The model under review builds one solid part; all positions refer to its coordinate system, in mm. Face numbers are marked on the shaded views. Round coordinates to 2 decimals unless told otherwise and drop trailing zeros. Write each loop counter-clockwise with the first axis right and the second up, starting at its lowest first coordinate (ties: lowest second). Pieces come first, ordered by that corner, then holes.
Item 1: Add section B-B (y = 2.4). Give the boundary of the cut face in (x, z), plus the area to 3 significant figures.
Item 2: Draft analysis for pull direction Z (two halves, no side actions). For the marked faces 1 and 2, state which applies: +Z half, -Z half, draft (parallel to the pull), parting line (faces both ways), or undercut.
Item 3: Clearance check with flat-ended pins moving along their axes: pin 1 Ø2 at (x, z) = (-5.5, -6.5) entering from -Y (3 decimals); pin 2 Ø2 at (x, z) = (-5.5, -8.5) entering from -Y; pin 3 Ø5 at (x, z) = (-12.82, 7.55) entering from +Y; pin 4 Ø1.5 at (x, y) = (4.5, 2.5) entering from -Z. State where each tip first meets the part, or that it passes through.
Item 4: To check wall thickness, follow L1, parallel to X at y = 0.75, z = 0; L2, parallel to Z at x = 0, y = 1.95; L3, parallel to Z at x = 1, y = 2.15. State the ranges of each line that lie inside material, in increasing order.
Item 5: Add section A-A (z = 0). Give the boundary of the cut face in (x, y), plus the area to 3 significant figures.
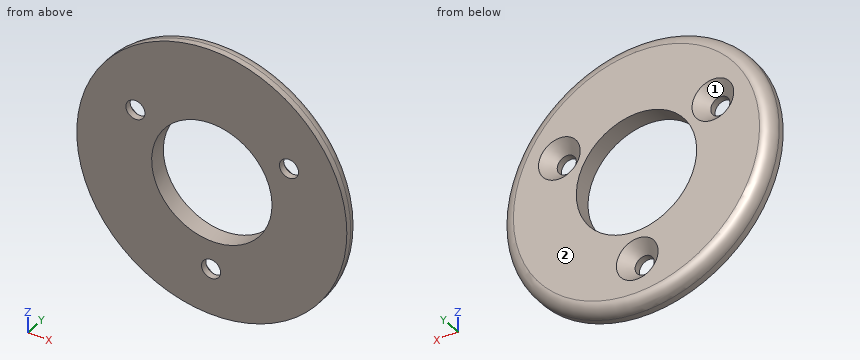
Autodesk Fusion 360 part; units mm, degrees
sketch "Sketch1" plane through (0, 0, 0) normal (0, 1, 0) x (1, 0, 0)
  circle A0 centre (0, 0) radius 22.661
extrude "Extrude1" add sketch "Sketch1" along normal blind 3
hole "Hole1" at (0, 3, 0) direction (0, -1, 0) diameter 20.2 depth 3 tip angle 180
hole "Hole2" at (-0.1263, 3, -14.8781) direction (0, -1, 0) diameter 3.2 depth 30 tip angle 180 countersink diameter 7 countersink angle 90
sketch "Sketch2" plane through (0, 0, 0) normal (0, 1, 0) x (1, 0, 0)
  circle A0 centre (0, 0) radius 15
  dimension "d9" = 30
pattern_circular "C-Pattern1" count 3 over 360 about axis through (0, 0, 0) along (0, 1, 0) of "Hole2"
fillet "Fillet1" radius 2 1 edges at (-21.1274, 3, 8.1946)
Numbers:
1. outline: circle Ø44.18 at (0, 0); hole circle Ø5.8 at (-12.82, 7.55); hole circle Ø20.2 at (0, 0); hole circle Ø5.8 at (-0.13, -14.88); hole circle Ø5.8 at (12.95, 7.33)
1. area: 1,130 mm2
2. face 1: undercut
2. face 2: draft
3. pin 1: passes through
3. pin 2: stops at y = 0
3. pin 3: stops at y = 2
3. pin 4: stops at z = -22.09
4. L1: x = -22.66 to -10.1, 10.1 to 22.66
4. L2: z = -22.42 to -17.32, -12.43 to -10.1, 10.1 to 22.42
4. L3: z = -22.27 to -17.28, -12.48 to -10.05, 10.05 to 22.27
5. outline: (-22.66, 0) - (-10.1, 0) - (-10.1, 3) - (-20.66, 3) arc R2 ccw to (-22.66, 1) - close; (10.1, 0) - (22.66, 0) - (22.66, 1) arc R2 ccw to (20.66, 3) - (10.1, 3) - close
5. area: 73.6 mm2
